For this review, take the finished solid that the model builds, in its own axes (mm). A direction names the side the tool comes from. Coordinates: 2 decimals unless noted, no trailing zeros. Loops run counter-clockwise (first coordinate to the right, second up) from the corner with the lowest first, then second, coordinate; pieces in that order, holes last. Notation, with made-up numbers: M 67.25,28 L 82.25,28 A13 cw 82.25,33 Z; hole C -34,61 d6. An arc over 180 degrees is marked long. Use one line per item in the form item = value.
```python
from build123d import *

# Parameters (mm, degrees)
F0_W     = 50.8
F0_H     = 50.8
F1_DEPTH = 7.62
F2_T     = -1.27
F3_W     = 1.27
F3_H     = 40.579203
F4_DEPTH = 6.35
F5_W     = 1.27
F5_H     = 17.874572
F5_H_2   = 22.697871
F6_DEPTH = 6.35
F7_W     = 1.27
F7_H     = 12.483831
F8_DEPTH = 6.35


with BuildPart() as f1:
    # F0 (on Top) → F1 (new body)
    with BuildSketch(Plane.XY):
        with Locations((25.4, 25.4)):
            Rectangle(F0_W, F0_H)
    extrude(amount=F1_DEPTH)

    # F2
    f2_openings = [f1.faces().sort_by_distance(p)[0] for p in [
        (25.4, 25.4, 7.62),
    ]]
    offset(amount=F2_T, openings=f2_openings)

    # F3 (on face) → F4 (join)
    with BuildSketch(Plane.XY.offset(1.27)):
        with Locations((10.990904, 21.559601)):
            Rectangle(F3_W, F3_H)
    extrude(amount=F4_DEPTH)

    # F5 (on Top) → F6 (join)
    with BuildSketch(Plane.XY):
        with Locations((22.204734, 40.288722)):
            Rectangle(F5_W, F5_H)
        with Locations((33.972504, 13.760585)):
            Rectangle(F5_W, F5_H_2)
    extrude(amount=F6_DEPTH)

    # F7 (on Top) → F8 (join)
    with BuildSketch(Plane.XY):
        with Locations((32.418778, 43.551543)):
            Rectangle(F7_W, F7_H)
    extrude(amount=F8_DEPTH)


solid = f1.part
```
1. Consider section D-D on y = 22.5. Write out the cut boundary in (x, z).
Computed values:
outline = M 0,0 L 50.8,0 L 50.8,7.62 L 49.53,7.62 L 49.53,1.27 L 34.61,1.27 L 34.61,6.35 L 33.34,6.35 L 33.34,1.27 L 11.63,1.27 L 11.63,7.62 L 10.36,7.62 L 10.36,1.27 L 1.27,1.27 L 1.27,7.62 L 0,7.62 Z
2. Consider section A-A on z = 3. Write out the cut boundary in (x, y).
Computed values:
outline = M 0,0 L 50.8,0 L 50.8,50.8 L 0,50.8 Z; M 21.57,31.35 L 22.84,31.35 L 22.84,49.23 L 21.57,49.23 Z; M 33.34,2.41 L 34.61,2.41 L 34.61,25.11 L 33.34,25.11 Z; hole M 1.27,1.27 L 10.36,1.27 L 10.36,41.85 L 11.63,41.85 L 11.63,1.27 L 49.53,1.27 L 49.53,49.53 L 33.05,49.53 L 33.05,37.31 L 31.78,37.31 L 31.78,49.53 L 1.27,49.53 Z
3. Wall thickness on line 1 along X through (y, z) = (34, 4.25); line 2 along X through (y, z) = (8, 1.5); line 3 along X through (y, z) = (27.5, 5.25): over which ranges is each line inside the solid? List them lowest first. Write a range as from..to.
Computed values:
line_1 = 0..1.27, 10.36..11.63, 21.57..22.84, 49.53..50.8
line_2 = 0..1.27, 10.36..11.63, 33.34..34.61, 49.53..50.8
line_3 = 0..1.27, 10.36..11.63, 49.53..50.8
4. For pin 1 Ø1 at (x, y) = (22.5, 36) entering from +Z, flat-tipped, find the tip position at first contact; note if it passes through.
Computed values:
pin_1 = 6.35
5. Tool access review of faces 1 (the face through (6, 1.27, 4)), 2 (the face through (25, 26, 0)): name each direction out of +Z, -Z, +X, -X, +Y, -Y from which nothing blocks a thin tool from reaching the whole face with its end or side.
Computed values:
face_1 = +Z
face_2 = -Z, +X, -X, +Y, -Y
6. Consider section B-B on x = 37.5. Write out the cut boundary in (y, z).
Computed values:
outline = M 0,0 L 50.8,0 L 50.8,7.62 L 49.53,7.62 L 49.53,1.27 L 1.27,1.27 L 1.27,7.62 L 0,7.62 Z
7. Draft analysis for pull direction Y (two halves, no side actions). For faces 3 (the face through (25, 50.8, 4)), 4 (the face through (34, 2.412, 4)), 5 (the face through (0, 25, 4)), state which applies: +Y half, -Y half, draft (parallel to the pull), parting line (faces both ways), or undercut.
Computed values:
face_3 = +Y half
face_4 = undercut
face_5 = draft
8. Consider section C-C on y = 42.5. Write out the cut boundary in (x, z), plus the area to 3 significant figures.
Computed values:
outline = M 0,0 L 50.8,0 L 50.8,7.62 L 49.53,7.62 L 49.53,1.27 L 33.05,1.27 L 33.05,6.35 L 31.78,6.35 L 31.78,1.27 L 22.84,1.27 L 22.84,6.35 L 21.57,6.35 L 21.57,1.27 L 1.27,1.27 L 1.27,7.62 L 0,7.62 Z
area = 93.5 mm2
